Autodesk Inventor part; units mm, degrees
ref_plane "YZ Plane" through (0, 0, 0) normal (1, 0, 0) x (0, 1, 0)
ref_plane "XZ Plane" through (0, 0, 0) normal (0, 1, 0) x (-1, 0, 0)
ref_plane "XY Plane" through (0, 0, 0) normal (0, 0, 1) x (1, 0, 0)
sketch "Эскиз1" plane through (0, 0, 0) normal (0, 0, 1) x (1, 0, 0)
  line L0 (-62.5, 20) -> (62.5, 20)
  line L1 (62.5, 20) -> (62.5, -20)
  line L2 (62.5, -20) -> (-62.5, -20)
  line L3 (-62.5, -20) -> (-62.5, 20)
  line L4 (-62.5, 20) -> (62.5, -20) construction
  line L5 (62.5, 20) -> (-62.5, -20) construction
  point P0 (0, 0)
  dimension "d0" = 125
  dimension "d1" = 40
extrude "Выдавливание1" add sketch "Эскиз1" along normal blind 4
sketch "Эскиз2" plane through (0, 0, 4) normal (0, 0, 1) x (1, 0, 0)
  circle A0 centre (-58.5, 16) radius 1.6
  line L0 (62.5, 20) -> (-62.5, 20)
  line L1 (-62.5, 20) -> (-62.5, -20)
  line L2 (-62.5, -20) -> (62.5, -20) construction
  line L3 (0, -20) -> (0, 0) construction
  line L4 (62.5, 0) -> (0, 0) construction
  circle A1 centre (58.5, 16) radius 1.6
  circle A2 centre (-58.5, -16) radius 1.6
  circle A3 centre (58.5, -16) radius 1.6
  dimension "d4" = 3.2
  dimension "d5" = 4
  dimension "d6" = 4
extrude "Выдавливание2" cut sketch "Эскиз2" against normal blind 4
sketch "Эскиз3" plane through (0, 0, 0) normal (0, 0, -1) x (-1, 0, 0)
  circle A0 centre (-49.5, 15.5) radius 1.5
  circle A1 centre (-49.5, -17) radius 1.5
  circle A2 centre (12.5, 15.5) radius 1.5
  circle A3 centre (12.5, -17) radius 1.5
  line L0 (29.7154, -12) -> (22.7872, 0)
  line L1 (22.7872, 0) -> (29.7154, 12)
  line L2 (29.7154, 12) -> (43.5718, 12)
  line L3 (43.5718, 12) -> (50.5, 0)
  line L4 (50.5, 0) -> (43.5718, -12)
  line L5 (43.5718, -12) -> (29.7154, -12)
  line L6 (-62.5, 20) -> (62.5, 20)
  line L7 (62.5, -20) -> (-62.5, -20)
  line L8 (-5.2128, 0) -> (-12.141, -12)
  line L9 (-12.141, -12) -> (-25.9974, -12)
  line L10 (-25.9974, -12) -> (-32.9256, 0)
  line L11 (-32.9256, 0) -> (-25.9974, 12)
  line L12 (-25.9974, 12) -> (-12.141, 12)
  line L13 (-12.141, 12) -> (-5.2128, 0)
  line L14 (62.5, 20) -> (62.5, -20)
  point P0 (0, 0)
  point P1 (36.6436, 0)
  point P2 (-19.0692, 0)
  point P3 (-19.0692, -12)
  point P4 (62.5, 0)
  dimension "d10" = 8
  dimension "d11" = 8
  dimension "d12" = 8
  dimension "d13" = 8
  dimension "d14" = 28
  dimension "d15" = 12
extrude "Выдавливание3" cut sketch "Эскиз3" against normal blind 4
properties part number "для_стаба"
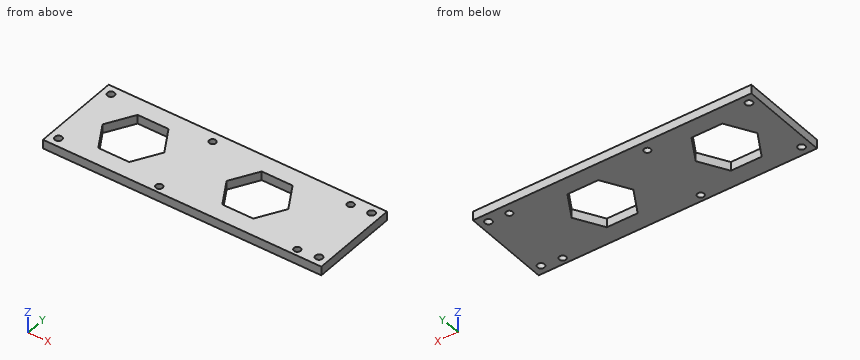
Can you work these out from the model? Positions are in its coordinate system, mm. Coordinates: 2 decimals unless noted, no trailing zeros. Loops run counter-clockwise (first coordinate to the right, second up) from the corner with the lowest first, then second, coordinate; pieces in that order, holes last. Notation, with made-up numbers: M 57.25,67.5 L 68.25,67.5 A22 cw 68.25,74.5 Z; hole C -11.75,25 d5. An arc over 180 degrees is marked long. Return JSON: item names as keys, results as strings. Group by question number.
Item 1: I'm going to push a flat-ended pin straight in: pin 1 Ø2.5 at (x, y) = (49.5, -17) entering from +Z. Where does the tip first touch, or does it pass through?
Item 2: If I drill on L1, parallel to Y at x = -58.5, z = 2.8; L2, parallel to X at y = 0, z = 2.35; L3, parallel to Y at x = -12.5, z = 1.9, over which ranges is the centre line in solid material (lowest first)? Write a range as from..to.
Item 3: Imagine slicing it at B-B (z = 0.6). Give the number of separate pieces and of enclosed holes in the cut face, and give its area (3 significant figures).
Item 4: Imagine slicing it at A-A (x = 58.5). Please give me the cut outline in (y, z).
Item 5: Imagine slicing it at D-D (y = 3). Please give me the cut outline in (x, z).
Item 6: Imagine slicing it at C-C (x = -34.5). Please give me the cut outline in (y, z), and give its area (3 significant figures).
Verdict:
{
 "1": {"pin 1": "passes through"},
 "2": {"L1": "y = -20..-17.6, -14.4..14.4, 17.6..20", "L2": "x = -62.5..-50.5, -22.79..5.21, 32.93..62.5", "L3": "y = -20..-18.5, -15.5..14, 17..20"},
 "3": {"separate pieces": "1", "enclosed holes": "10", "area": "3,940 mm^2"},
 "4": {"outline": "M -20,0 L -17.6,0 L -17.6,4 L -20,4 Z; M -14.4,0 L 14.4,0 L 14.4,4 L -14.4,4 Z; M 17.6,0 L 20,0 L 20,4 L 17.6,4 Z"},
 "5": {"outline": "M -62.5,0 L -48.77,0 L -48.77,4 L -62.5,4 Z; M -24.52,0 L 6.94,0 L 6.94,4 L -24.52,4 Z; M 31.19,0 L 62.5,0 L 62.5,4 L 31.19,4 Z"},
 "6": {"outline": "M -20,0 L -12,0 L -12,4 L -20,4 Z; M 12,0 L 20,0 L 20,4 L 12,4 Z", "area": "64.0 mm^2"}
}
